Build history of the part. All positions in model axes, mm. Face numbers are marked on the shaded views. A direction names the side the tool comes from. Round coordinates to 2 decimals unless told otherwise and drop trailing zeros. Write each loop counter-clockwise with the first axis right and the second up, starting at its lowest first coordinate (ties: lowest second). Pieces come first, ordered by that corner, then holes.
1) Which spindle directions (+Z, -Z, +X, -X, +Y, -Y) get a long thin tool onto all of the face, cutting with end or side? Do the marked faces 1, 2 and 3. Say none if no direction does.
2) Saw through at B-B (z = -15). Write the cut outline in (x, y).
3) Saw through at D-D (z = -10). Write the cut outline in (x, y), plus the area to 3 significant figures.
4) Pull direction Y, two halves, no side cores. Call the marked faces 4, 5 and 6: +Y half, -Y half, draft (parallel to the pull), parting line (faces both ways), or undercut.
5) Saw through at C-C (z = -4). Write the cut outline in (x, y), plus the area to 3 significant figures.
6) Flat gauge pins, fed straight in: pin 1 (0.8 mm diameter, centred on x = -14.5, z = -15, fed in from +Y); pin 2 (6 mm diameter, centred on x = -11.5, y = -1.5, fed in from +Z); pin 3 (0.5 mm diameter, centred on x = 8, y = 13, fed in from +Z); pin 4 (6.5 mm diameter, centred on y = 13.5, z = -15, fed in from -X). Where does each tip first touch, or does it go through?
7) Wall check: probe 1 along X at (y, z) = (8.5, -15.25); probe 2 along Z at (x, y) = (-8.25, 13.5); probe 3 along X at (y, z) = (10.5, -8). Give the ranges that are in metal, low to high.
8) Saw through at A-A (x = 0). Write the cut outline in (y, z), plus the area to 3 significant figures.
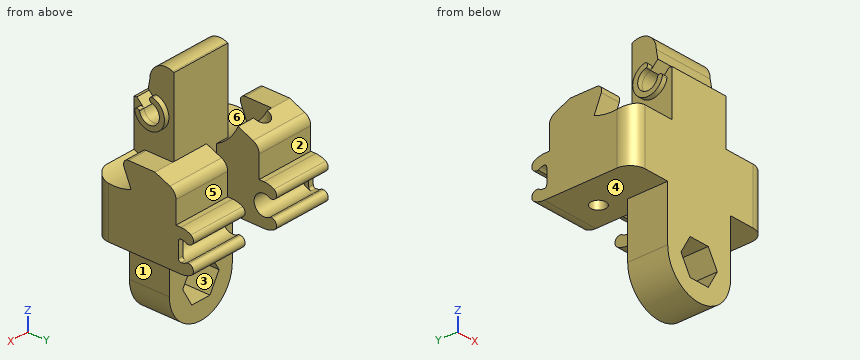
from build123d import *
from build123d.topology import SkipClean

# Parameters (mm, degrees)
BOSS_EXTRUDE1_DEPTH      = 6
BOSS_EXTRUDE2_DEPTH      = 7
SKETCH6_R                = 7
BOSS_EXTRUDE3_DEPTH      = 18
BOSS_EXTRUDE4_DEPTH      = 8
BOSS_EXTRUDE4_DEPTH_BACK = 8
SKETCH7_R                = 4.5
CUT_EXTRUDE2_DEPTH       = 5
CUT_EXTRUDE4_START       = -5
CUT_EXTRUDE4_DEPTH       = 5
BOSS_EXTRUDE6_DEPTH      = 1
FILLET3_R                = 0.5
FILLET3_OF_MIRROR1_R     = 0.5
BOSS_EXTRUDE5_DEPTH      = 15
SKETCH20_W               = 7
SKETCH20_H               = 38
CUT_EXTRUDE7_DEPTH       = 42.913087917
FILLET1_START            = -6
FILLET1_DEPTH            = 12
FILLET2_R                = 1
CUT_EXTRUDE8_DEPTH       = 42.560578801
BOSS_EXTRUDE7_DEPTH      = 1
FILLET4_R                = 0.5
FILLET4_OF_MIRROR2_R     = 0.5
FILLET5_R                = 3
FILLET7_R                = 2
CUT_SWEEP1_PROFILE_R     = 1.5
BOSS_EXTRUDE8_DEPTH      = 4
FILLET8_R                = 1
FILLET8_OF_MIRROR3_R     = 1


with BuildPart() as part:
    # Sketch3 → Boss-Extrude1 (new, symmetric)
    with BuildSketch(Plane(origin=(0, 0, 0), x_dir=(0, 0, -1), z_dir=(1, 0, 0))):
        with BuildLine():
            ThreePointArc((2, 0), (1.51090791, -1.310403483), (0.282842712, -1.979898987))
            Line((0.282842712, -1.979898987), (-1.13137085, -3.39411255))
            Line((-1.13137085, -3.39411255), (-0.81880413, -5.166766505))
            Line((-0.81880413, -5.166766505), (-3.807139593, -8.155101968))
            ThreePointArc((-3.807139593, -8.155101968), (4.834032667, -7.591582718), (9, 0))
            ThreePointArc((9, 0), (-1.949882341, 8.7862369), (-8.155101968, -3.807139593))
            Line((-8.155101968, -3.807139593), (-5.166766505, -0.81880413))
            Line((-5.166766505, -0.81880413), (-3.39411255, -1.13137085))
            Line((-3.39411255, -1.13137085), (-1.979898987, 0.282842712))
            ThreePointArc((-1.979898987, 0.282842712), (0.14177804, 1.994968418), (2, 0))
        make_face()
    extrude(amount=BOSS_EXTRUDE1_DEPTH, both=True)

    # Sketch5 → Boss-Extrude2 (add, symmetric)
    with BuildSketch(Plane(origin=(0, 0, 0), x_dir=(0, 0, -1), z_dir=(1, 0, 0))):
        with BuildLine():
            Line((0, 9), (29.855960009, 9))
            Line((29.855960009, 9), (29.855960009, -9))
            Line((29.855960009, -9), (0, -9))
            ThreePointArc((0, -9), (9, 0), (0, 9))
        make_face()
    extrude(amount=BOSS_EXTRUDE2_DEPTH, both=True)

    # Sketch6 → Boss-Extrude3 (add)
    with BuildSketch(Plane(origin=(0, 9, 0), x_dir=(1, 0, 0), z_dir=(0, 1, 0))):
        with Locations((0, 29.855960009)):
            Circle(SKETCH6_R)
    extrude(amount=-BOSS_EXTRUDE3_DEPTH)

    # Sketch7 → Boss-Extrude4 (add, two sides: drawn at the far end of the back side and taken through both)
    with BuildSketch(Plane(origin=(0, 0, 0), x_dir=(1, 0, 0), z_dir=(0, 1, 0)).offset(-BOSS_EXTRUDE4_DEPTH_BACK)):
        with Locations((0, 29.855960009)):
            Circle(SKETCH7_R)
    extrude(amount=BOSS_EXTRUDE4_DEPTH + BOSS_EXTRUDE4_DEPTH_BACK)

    # Sketch8 → Cut-Extrude2 (cut)
    with BuildSketch(Plane(origin=(0, 9, 0), x_dir=(1, 0, 0), z_dir=(0, 1, 0))):
        with BuildLine():
            Line((6, -9), (6, 0))
            Line((6, 0), (7, 0))
            Line((7, 0), (7, 29.855960009))
            ThreePointArc((7, 29.855960009), (0, 36.855960009), (-7, 29.855960009))
            Line((-7, 29.855960009), (-7, 0))
            Line((-7, 0), (-6, 0))
            Line((-6, 0), (-6, -9))
            Line((-6, -9), (6, -9))
        make_face()
    extrude(amount=-CUT_EXTRUDE2_DEPTH, mode=Mode.SUBTRACT)

    # Sketch9 → Cut-Extrude4 (cut)
    with BuildSketch(Plane.XZ.offset(9).offset(CUT_EXTRUDE4_START)):
        with BuildLine():
            Line((6, 0), (6, 9))
            Line((6, 9), (-6, 9))
            Line((-6, 9), (-6, 0))
            Line((-6, 0), (-7, 0))
            Line((-7, 0), (-7, -29.855960009))
            ThreePointArc((-7, -29.855960009), (0, -36.855960009), (7, -29.855960009))
            Line((7, -29.855960009), (7, 0))
            Line((7, 0), (6, 0))
        make_face()
    extrude(amount=CUT_EXTRUDE4_DEPTH, mode=Mode.SUBTRACT)

    # Sketch24 → Boss-Extrude6 (add)
    with SkipClean():  # the faces are left unmerged after this step: merging them gives an invalid solid
        with BuildSketch(Plane.ZY.offset(6)):
            with BuildLine():
                ThreePointArc((-0.282842712, -1.979898987), (-1.414213562, 1.414213562), (1.979898987, 0.282842712))
                Line((1.979898987, 0.282842712), (2.925806694, -0.663064995))
                ThreePointArc((2.925806694, -0.663064995), (2.981393976, -0.333601496), (3, 0))
                ThreePointArc((3, 0), (-2.344055778, 1.872272018), (0.663064995, -2.925806694))
                Line((0.663064995, -2.925806694), (-0.282842712, -1.979898987))
            make_face()
        boss_extrude6 = extrude(amount=BOSS_EXTRUDE6_DEPTH)

    # Fillet3
    # the kernel refuses this fillet: 0.5 mm, written as the material it takes off along each edge
    with BuildSketch(Plane(origin=(-6, -0.663064995, 2.925806694), x_dir=(0, 0.9999849386062066, 0.005488402385122609), z_dir=(-1, 0, 0))) as fillet3_piece_1:
        with BuildLine():
            CenterArc((1.186161173, 0.488233633), FILLET3_R, 135.314463872, 147.140119621)
            Line((0.830672664, 0.839841255), (0, 0))
            ThreePointArc((0, 0), (0.646997003, -0.070598205), (1.293994007, 0))
        make_face()
    extrude(amount=4.234985017, mode=Mode.SUBTRACT)
    with BuildSketch(Plane(origin=(-6, -2.925806694, 0.663064995), x_dir=(0, -0.005488402385198552, -0.9999849386062063), z_dir=(-1, 0, 0))) as fillet3_piece_2:
        with BuildLine():
            CenterArc((1.186161173, -0.488233633), FILLET3_R, 77.545416507, 147.140119621)
            Line((0.830672664, -0.839841255), (0, 0))
            ThreePointArc((0, 0), (0.646997003, 0.070598205), (1.293994007, 0))
        make_face()
    extrude(amount=4.234985017, mode=Mode.SUBTRACT)

    # Mirror1: Boss-Extrude6 across plane
    add(boss_extrude6.mirror(Plane(origin=(0, 0, 0), x_dir=(0, 0, 1), z_dir=(1, 0, 0))))

    # Fillet3 of Mirror1
    # the kernel refuses this fillet: 0.5 mm, written as the material it takes off along each edge
    with BuildSketch(Plane(origin=(6, -0.663064995, 2.925806694), x_dir=(0, 0.7071067811865444, -0.7071067811865507), z_dir=(1, 0, 0))) as fillet3_of_mirror1_piece_1:
        with BuildLine():
            CenterArc((1.181249511, 0.5), FILLET3_OF_MIRROR1_R, 122.859880379, 147.140119621)
            ThreePointArc((0.909956312, 0.92), (0.404784455, 0.509645734), (0, 0))
            Line((0, 0), (1.181249511, 0))
        make_face()
    extrude(amount=4.234985017, mode=Mode.SUBTRACT)
    with BuildSketch(Plane(origin=(6, -2.925806694, 0.663064995), x_dir=(0, 0.7071067811865442, -0.7071067811865509), z_dir=(1, 0, 0))) as fillet3_of_mirror1_piece_2:
        with BuildLine():
            CenterArc((1.181249511, -0.5), FILLET3_OF_MIRROR1_R, 90, 147.140119621)
            ThreePointArc((0.909956312, -0.92), (0.404784455, -0.509645734), (0, 0))
            Line((0, 0), (1.181249511, 0))
        make_face()
    extrude(amount=4.234985017, mode=Mode.SUBTRACT)

    # Sketch10 → Boss-Extrude5 (add, symmetric)
    with BuildSketch(Plane(origin=(0, 0, 0), x_dir=(0, 0, -1), z_dir=(1, 0, 0))):
        with BuildLine():
            ThreePointArc((8.062257748, -4), (9, 0), (8.062257748, 4))
            Line((8.062257748, 4), (19, 4))
            Line((19, 4), (19, -4))
            Line((19, -4), (8.062257748, -4))
        make_face()
        with BuildLine():
            Line((13.4, 17.166060556), (13.4, 14.7))
            ThreePointArc((13.4, 14.7), (15, 11.5), (16.6, 14.7))
            Line((16.6, 14.7), (16.6, 17.166060556))
            ThreePointArc((16.6, 17.166060556), (18.346640106, 15.69089023), (19, 13.5))
            Line((19, 13.5), (19, 4))
            Line((19, 4), (8.062257748, 4))
            ThreePointArc((8.062257748, 4), (6.173062485, 6.549297638), (3.516580156, 8.284543681))
            Line((3.516580156, 8.284543681), (5.305935203, 12.5))
            Line((5.305935203, 12.5), (11, 12.5))
            Line((11, 12.5), (11, 13.5))
            ThreePointArc((11, 13.5), (11.653359894, 15.69089023), (13.4, 17.166060556))
        make_face()
    extrude(amount=BOSS_EXTRUDE5_DEPTH, both=True)

    # Sketch20 → Cut-Extrude7 (cut, through all)
    with BuildSketch(Plane(origin=(0, 4, 0), x_dir=(1, 0, 0), z_dir=(0, 1, 0))):
        Rectangle(SKETCH20_W, SKETCH20_H)
    extrude(amount=CUT_EXTRUDE7_DEPTH, mode=Mode.SUBTRACT)

    # Fillet1: read off the stored shape, not the designer's step
    # Fillet1 outline → Fillet1 (cut)
    with BuildSketch(Plane.YZ.offset(FILLET1_START)):
        with BuildLine():
            ThreePointArc((-0.81880413, 5.166766505), (0.666331593, 7.940128227), (3.804881491, 8.156155764))
            ThreePointArc((3.804881491, 8.156155764), (-0.001245944, 8.999999913), (-3.807139593, 8.155101968))
            Line((-3.807139593, 8.155101968), (-0.81880413, 5.166766505))
        make_face()
    extrude(amount=FILLET1_DEPTH, mode=Mode.SUBTRACT)

    # Fillet2
    fillet2_edges = [part.edges().sort_by_distance(p)[0] for p in [
        (9.25, 17.166060556, -16.6),
        (9.25, 17.166060556, -13.4),
        (-9.25, 17.166060556, -13.4),
        (-9.25, 17.166060556, -16.6),
    ]]
    fillet(fillet2_edges, radius=FILLET2_R)

    # Sketch23 → Cut-Extrude8 (cut, through all)
    with BuildSketch(Plane(origin=(0, 4, 0), x_dir=(1, 0, 0), z_dir=(0, 1, 0))):
        Polygon((4.041451884, 29.855960009), (2.020725942, 33.355960009), (-2.020725942, 33.355960009), (-4.041451884, 29.855960009), (-2.020725942, 26.355960009), (2.020725942, 26.355960009), align=None)
    extrude(amount=-CUT_EXTRUDE8_DEPTH, mode=Mode.SUBTRACT)

    # Sketch25 → Boss-Extrude7 (add)
    with BuildSketch(Plane(origin=(15, 0, 0), x_dir=(0, 0, -1), z_dir=(1, 0, 0))):
        with BuildLine():
            Line((16.936491673, 13), (13.063508327, 13))
            ThreePointArc((13.063508327, 13), (15, 11.5), (16.936491673, 13))
        make_face()
    boss_extrude7 = extrude(amount=-BOSS_EXTRUDE7_DEPTH)

    # Fillet4
    fillet4_edges = [part.edges().sort_by_distance(p)[0] for p in [
        (14.5, 13, -13.063508327),
        (14.5, 13, -16.936491673),
    ]]
    fillet(fillet4_edges, radius=FILLET4_R)

    # Mirror2: Boss-Extrude7 across plane
    add(boss_extrude7.mirror(Plane(origin=(0, 0, 0), x_dir=(0, 0, 1), z_dir=(1, 0, 0))))

    # Fillet4 of Mirror2
    fillet4_of_mirror2_edges = [part.edges().sort_by_distance(p)[0] for p in [
        (-14.5, 13, -13.063508327),
        (-14.5, 13, -16.936491673),
    ]]
    fillet(fillet4_of_mirror2_edges, radius=FILLET4_OF_MIRROR2_R)

    # Fillet5
    fillet5_edges = [part.edges().sort_by_distance(p)[0] for p in [
        (15, -4, -13.531128874),
        (-15, -4, -13.531128874),
    ]]
    fillet(fillet5_edges, radius=FILLET5_R)

    # Fillet7
    fillet7_edges = [part.edges().sort_by_distance(p)[0] for p in [
        (9.25, 12.5, -5.305935203),
        (-9.25, 12.5, -5.305935203),
    ]]
    fillet(fillet7_edges, radius=FILLET7_R)

    # Cut-Sweep1: sweep along a path in Sketch27
    with BuildLine(Plane.ZY.offset(8.5)) as cut_sweep1_path:
        Line((0, 8.5), (-25.421416279, 8.5))
    # Cut-Sweep1 profile (on start of the path) → Cut-Sweep1 (sweep, cut)
    with BuildSketch(Plane(origin=(-8.5, 8.5, 0), x_dir=(0, -1, 0), z_dir=(0, 0, -1))):
        Circle(CUT_SWEEP1_PROFILE_R)
    sweep(path=cut_sweep1_path.line, mode=Mode.SUBTRACT)

    # Sketch28 → Boss-Extrude8 (add)
    with BuildSketch(Plane(origin=(15, 0, 0), x_dir=(0, 0, -1), z_dir=(1, 0, 0))):
        with BuildLine():
            Line((3.516580156, 1.492699716), (8.284543681, 3.516580156))
            ThreePointArc((8.284543681, 3.516580156), (6.363961031, 6.363961031), (3.516580156, 8.284543681))
            Line((3.516580156, 8.284543681), (3.516580156, 1.492699716))
        make_face()
    boss_extrude8 = extrude(amount=-BOSS_EXTRUDE8_DEPTH)

    # Fillet8
    fillet8_edges = [part.edges().sort_by_distance(p)[0] for p in [
        (13, 1.492699716, -3.516580156),
    ]]
    fillet(fillet8_edges, radius=FILLET8_R)

    # Mirror3: Boss-Extrude8 across plane
    add(boss_extrude8.mirror(Plane(origin=(0, 0, 0), x_dir=(0, 0, 1), z_dir=(1, 0, 0))))

    # Fillet8 of Mirror3
    fillet8_of_mirror3_edges = [part.edges().sort_by_distance(p)[0] for p in [
        (-13, 1.492699716, -3.516580156),
    ]]
    fillet(fillet8_of_mirror3_edges, radius=FILLET8_OF_MIRROR3_R)


solid = part.part
Evaluation:
1. face 1: -Z, +X, +Y, -Y
1. face 2: +Z, +X, -X, +Y
1. face 3: +Y, -Y
2. outline: (-15, -1) arc R3 ccw to (-12, -4) - (12, -4) arc R3 ccw to (15, -1) - (15, 13) - (14, 13) - (14, 11.5) - (3.5, 11.5) - (3.5, 4) - (-3.5, 4) - (-3.5, 11.5) - (-14, 11.5) - (-14, 13) - (-15, 13) - close; hole circle Ø3 at (-8.5, 8.5)
3. outline: (-15, -1) arc R3 ccw to (-12, -4) - (12, -4) arc R3 ccw to (15, -1) - (15, 12.5) - (3.5, 12.5) - (3.5, 4) - (-3.5, 4) - (-3.5, 12.5) - (-15, 12.5) - close; hole circle Ø3 at (-8.5, 8.5)
3. area: 425 mm2
4. face 4: draft
4. face 5: +Y half
4. face 6: undercut
5. outline: (-15, 2.15) - (-11, 2.15) - (-11, 8.06) - (-9.93, 8.06) arc R1.5 cw to (-9.68, 9.42) - (-15, 9.42) - close; (-7.32, 9.42) arc R1.5 cw to (-7.07, 8.06) - (-3.5, 8.06) - (-3.5, 9.42) - close; (-6, -4) - (6, -4) - (6, 4) - (-6, 4) - close; (3.5, 8.06) - (11, 8.06) - (11, 2.15) - (15, 2.15) - (15, 9.42) - (3.5, 9.42) - close
5. area: 171 mm2
6. pin 1: stops at y = 13
6. pin 2: stops at z = -8.06
6. pin 3: stops at z = -11
6. pin 4: stops at x = -15
7. probe 1: x = -15 to -10, -7 to -3.5, 3.5 to 15
7. probe 2: z = -19 to -17, -13 to -11
7. probe 3: x = -15 to -3.5, 3.5 to 15
8. outline: (-4, -36.86) - (4, -36.86) - (4, -33.36) - (-4, -33.36) - close; (-4, -26.36) - (4, -26.36) - (4, 8.06) arc R9 ccw to (3.8, 8.16) arc R3.25 ccw to (-0.82, 5.17) - (-1.13, 3.39) - (0.28, 1.98) arc R2 cw (long way) to (-1.98, -0.28) - (-3.39, 1.13) - (-4, 1.02) - close
8. area: 267 mm2
